Autodesk Inventor part; units mm, degrees
ref_plane "YZ Plane" through (0, 0, 0) normal (1, 0, 0) x (0, 1, 0)
ref_plane "XZ Plane" through (0, 0, 0) normal (0, 1, 0) x (-1, 0, 0)
ref_plane "XY Plane" through (0, 0, 0) normal (0, 0, 1) x (1, 0, 0)
sketch "Sketch1" plane through (0, 0, 0) normal (1, 0, 0) x (0, 1, 0)
  line L0 (8, 10) -> (-8, 10)
  line L1 (-8, 10) -> (-8, -140)
  line L2 (-8, -140) -> (8, -140)
  line L3 (8, -140) -> (8, 10)
  point P0 (0, 0)
  dimension "d0" = 16
  dimension "d1" = 8
  dimension "d2" = 10
  dimension "d3" = 150
extrude "Extrusion1" add sketch "Sketch1" along normal blind 10
sketch "Sketch2" plane through (10, 0, 0) normal (1, 0, 0) x (0, 0, -1)
  point P0 (0, 0)
  point P1 (0, 0)
hole "Hole1" at (10, 0, 0) direction (-1, 0, 0) diameter 10 depth 22 tip angle 118
sketch "Sketch3" plane through (10, 0, 0) normal (1, 0, 0) x (0, 0, -1)
  point P0 (0, 0)
  point P1 (70, 0)
  dimension "d20" = 0
  dimension "d21" = 70
hole "Hole2" at (10, 0, -70) direction (-1, 0, 0) diameter 10 depth 22 tip angle 118
properties part number "Haste"
CAD build for the part. Positions are in the model's coordinates, mm. Round coordinates to 2 decimals unless told otherwise and drop trailing zeros. Order: outer loops, then holes, each group sorted by start corner. A loop starts at its lowest first (then second) coordinate and runs counter-clockwise, first axis right, second up. Notation, with made-up numbers: (-28, 5) - (19, 5) arc R11 cw to (19, 15) - close; hole circle Ø7 at (-16.75, 61). An arc over 180 degrees is marked (long way). Return JSON: item names as keys, results as strings.
(1) Cut at A-A (z = -70). Give the cut face in (x, y), then the cut area to 3 significant figures.
Answer key:
{"outline": "(0, -8) - (10, -8) - (10, -5) - (0, -5) - close; (0, 5) - (10, 5) - (10, 8) - (0, 8) - close", "area": "60.0 mm^2"}
(2) Pull direction Y, two halves, no side cores. Call faces 1 (the face through (5, 8, -66)), 2 (the face through (4.93, 4.88, 1.08)), 3 (the face through (5, 0, 10)), 4 (the face through (4.93, 1.915, -74.619)): +Y half, -Y half, draft (parallel to the pull), parting line (faces both ways), or undercut.
Answer key:
{"face 1": "+Y half", "face 2": "undercut", "face 3": "draft", "face 4": "undercut"}
(3) Cut at C-C (x = 8). Give the cut face in (y, z), then the cut area to 3 significant figures.
Answer key:
{"outline": "(-8, -140) - (8, -140) - (8, 10) - (-8, 10) - close; hole circle Ø10 at (0, -70); hole circle Ø10 at (0, 0)", "area": "2,240 mm^2"}
(4) Pin check, flat tip, straight feed: pin 1 Ø6 at (y, z) = (0, 0) entering from -X. Stop position of the tip, or through.
Answer key:
{"pin 1": "passes through"}
(5) Wall check: probe 1 along Z at (x, y) = (5.25, 0); probe 2 along Y at (x, z) = (4.5, -70); probe 3 along Z at (x, y) = (6, -1). Give the ranges that are in metal, low to high. Write a range as from..to.
Answer key:
{"probe 1": "z = -140..-75, -65..-5, 5..10", "probe 2": "y = -8..-5, 5..8", "probe 3": "z = -140..-74.9, -65.1..-4.9, 4.9..10"}
(6) Cut at B-B (y = 0). Give the cut face in (x, z).
Answer key:
{"outline": "(0, -140) - (10, -140) - (10, -75) - (0, -75) - close; (0, -65) - (10, -65) - (10, -5) - (0, -5) - close; (0, 5) - (10, 5) - (10, 10) - (0, 10) - close"}
